Part model, mm, in its own coordinate system. Round coordinates to 2 decimals unless told otherwise and drop trailing zeros. Order: outer loops, then holes, each group sorted by start corner. A loop starts at its lowest first (then second) coordinate and runs counter-clockwise, first axis right, second up. Notation, with made-up numbers: (21, 57.25) -> (29, 57.25) arc R18 ccw to (29, 72.25) -> close; hole circle Ø8 at (21, 7). An arc over 180 degrees is marked (long way). Answer as a JSON object with one key per item and string values. Group by question number.
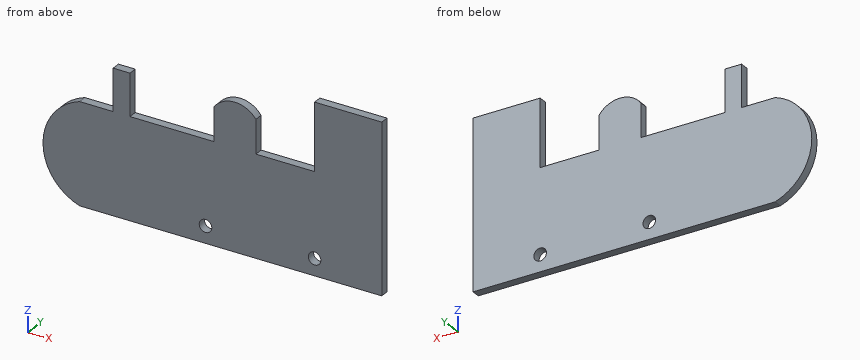
```python
from build123d import *

# Parameters (mm, degrees)
F0_W     = 80
F0_H     = 80
F0_W_2   = 20
F0_H_2   = 50
F0_W_3   = 50
F0_H_3   = 40
F1_DEPTH = 10
F2_R     = 7.5
F3_DEPTH = 10.001


with BuildPart() as f1:
    # F0 (on Front) → F1 (new body)
    with BuildSketch(Plane.XZ):
        Polygon((0, 120), (0, 0), (360, 0), (360, 120), (280, 120), (210, 120), (160, 120), (60, 120), (40, 120), align=None)
        with BuildLine():
            ThreePointArc((0, 120), (-43.622246, 60), (0, 0))
            Line((0, 0), (0, 120))
        make_face()
        with Locations((320, 160)):
            Rectangle(F0_W, F0_H)
        with Locations((50, 145)):
            Rectangle(F0_W_2, F0_H_2)
        with Locations((185, 140)):
            Rectangle(F0_W_3, F0_H_3)
        with BuildLine():
            Line((160, 160), (210, 160))
            ThreePointArc((210, 160), (185, 172.599857), (160, 160))
        make_face()
    extrude(amount=F1_DEPTH)

    # F2 (on face) → F3 (cut, through all)
    with BuildSketch(Plane.XZ.offset(10)):
        with Locations((150, 20)):
            Circle(F2_R)
        with Locations((280, 20)):
            Circle(F2_R)
    extrude(amount=-F3_DEPTH, mode=Mode.SUBTRACT)


solid = f1.part
```
Q1. Drop flat-ended pins along their axis: pin 1 Ø2 at (x, y) = (38.5, -6.5) entering from +Z; pin 2 Ø5 at (y, z) = (-4, 156) entering from -X. Give the stop position or say it passes through.
Q2. Band-saw the part on D-D (z = 183). List the corners of the cut face in (x, y), plus the area to 3 significant figures.
Q3. Band-saw the part on A-A (x = 150). List the corners of the cut face in (y, z).
Q4. Wall check: line 1 (X direction, y = -9, z = 151); line 2 (Z direction, x = 150, y = -1.75); line 3 (Z direction, x = 172.5, y = -3.75). Give the ranges that are in metal, low to high. Write a range as [from, to].
Q5. Band-saw the part on B-B (y = -2.75). List the corners of the cut face in (x, z), plus the area to 3 significant figures.
Q6. Band-saw the part on C-C (z = 134.5). List the corners of the cut face in (x, y).
Completed:
{
 "1": {"pin 1": "z = 120", "pin 2": "x = 40"},
 "2": {"outline": "(280, -10) -> (360, -10) -> (360, 0) -> (280, 0) -> close", "area": "800 mm2"},
 "3": {"outline": "(-10, 0) -> (0, 0) -> (0, 12.5) -> (-10, 12.5) -> close; (-10, 27.5) -> (0, 27.5) -> (0, 120) -> (-10, 120) -> close"},
 "4": {"line 1": "[40, 60], [160, 210], [280, 360]", "line 2": "[0, 12.5], [27.5, 120]", "line 3": "[0, 169.98]"},
 "5": {"outline": "(0, 0) -> (360, 0) -> (360, 200) -> (280, 200) -> (280, 120) -> (210, 120) -> (210, 160) arc R31.1 ccw to (160, 160) -> (160, 120) -> (60, 120) -> (60, 170) -> (40, 170) -> (40, 120) -> (0, 120) arc R63.07 ccw to start; hole circle Ø15 at (150, 20); hole circle Ø15 at (280, 20)", "area": "56,500 mm2"},
 "6": {"outline": "(40, -10) -> (60, -10) -> (60, 0) -> (40, 0) -> close; (160, -10) -> (210, -10) -> (210, 0) -> (160, 0) -> close; (280, -10) -> (360, -10) -> (360, 0) -> (280, 0) -> close"}
}
